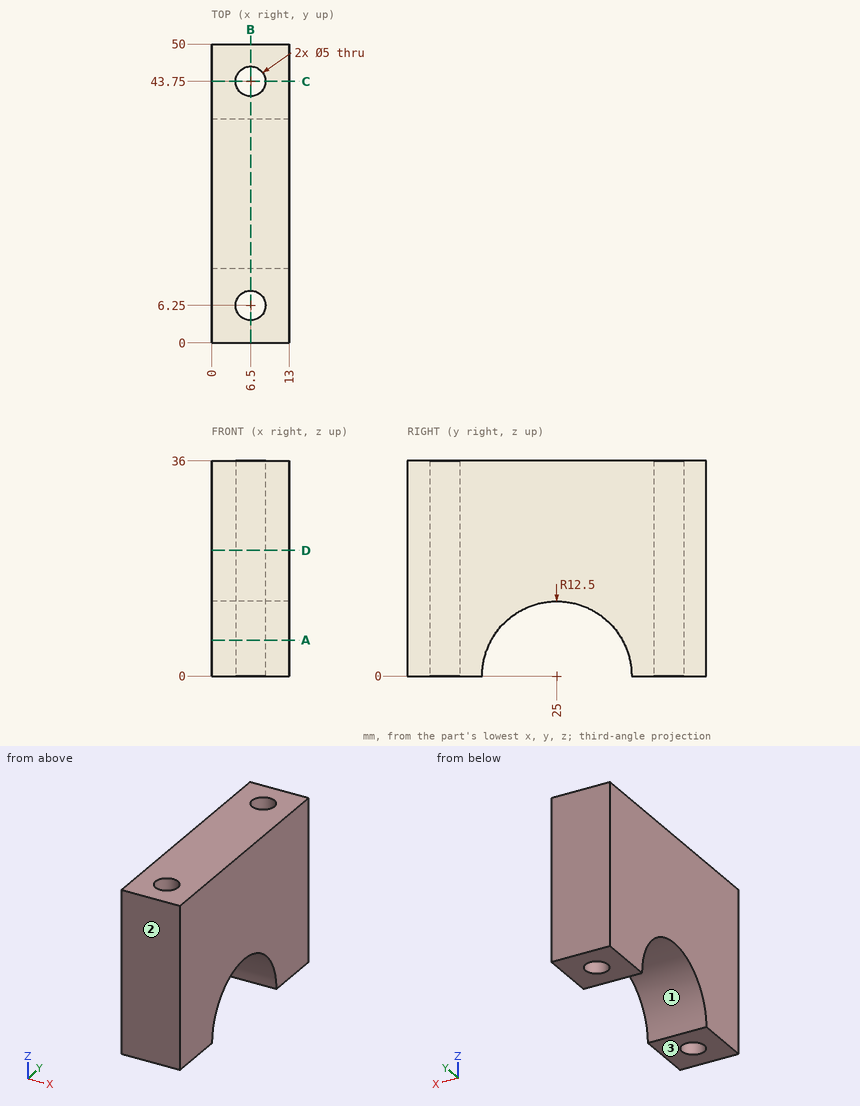
Answer from the drawing. Dimensions are ordinates in mm from the lowest x, y and z of the part. Give positions to 0.01 mm unless a question says otherwise; leave off trailing zeros. Loops run counter-clockwise (first coordinate to the right, second up) from the corner with the lowest first, then second, coordinate; pieces in that order, holes last. Notation, with made-up numbers: (-9, -11.5) -> (21, -11.5) arc R24 ccw to (21, 20.5) -> close; hole circle Ø2 at (-25.75, 35). An arc over 180 degrees is marked (long way). One line per question, with ' | ' between items. Start each with the question number.
1) Section A-A, the plane z = 6 is taken. Determine the outline of the cut face in (x, y).
2) Section C-C, the plane y = 43.75 is taken. Determine the outline of the cut face in (x, z).
3) Section B-B, the plane x = 6.5 is taken. Determine the outline of the cut face in (y, z).
4) Determine the mould class of the marked faces 1, 2 and 3 for opening direction Y: +Y half, -Y half, draft (parallel to the pull), parting line (faces both ways), or undercut.
5) Section D-D, the plane z = 21 is taken. Determine the outline of the cut face in (x, y), then the cut area to 3 significant figures.
6) This flat-tipped pin is pushed along its axis until it touches: pin 1 (3 mm diameter, centred on x = 2, y = 30.5, fed in from -Z). Where does it stop, or does it pass through?
7) Straight lines are drawn through the part: L1, parallel to Y at x = 6.5, z = 20.5; L2, parallel to X at y = 43.75, z = 16.5; L3, parallel to Y at x = 7.5, z = 7.5. For each, find the intervals that lie inside material, in ascending order.
Resolved:
1) outline: (0, 0) -> (13, 0) -> (13, 14.03) -> (0, 14.03) -> close; (0, 35.97) -> (13, 35.97) -> (13, 50) -> (0, 50) -> close; hole circle Ø5 at (6.5, 6.25); hole circle Ø5 at (6.5, 43.75)
2) outline: (0, 0) -> (4, 0) -> (4, 36) -> (0, 36) -> close; (9, 0) -> (13, 0) -> (13, 36) -> (9, 36) -> close
3) outline: (0, 0) -> (3.75, 0) -> (3.75, 36) -> (0, 36) -> close; (8.75, 0) -> (12.5, 0) arc R12.5 cw to (37.5, 0) -> (41.25, 0) -> (41.25, 36) -> (8.75, 36) -> close; (46.25, 0) -> (50, 0) -> (50, 36) -> (46.25, 36) -> close
4) face 1: undercut | face 2: -Y half | face 3: draft
5) outline: (0, 0) -> (13, 0) -> (13, 50) -> (0, 50) -> close; hole circle Ø5 at (6.5, 6.25); hole circle Ø5 at (6.5, 43.75) | area: 611 mm2
6) pin 1: z = 10.36
7) L1: 0 to 3.75, 8.75 to 41.25, 46.25 to 50 | L2: 0 to 4, 9 to 13 | L3: 0 to 3.96, 8.54 to 15, 35 to 41.46, 46.04 to 50
